Geometry: final body of the model. Coordinates: model frame, mm. Round coordinates to 2 decimals unless told otherwise and drop trailing zeros. Loops run counter-clockwise (first coordinate to the right, second up) from the corner with the lowest first, then second, coordinate; pieces in that order, holes last. Notation, with made-up numbers: (19.25, 2.25) -> (50.25, 2.25) arc R37 cw to (50.25, 38.25) -> close; hole circle Ø1 at (-6, 28). An arc over 180 degrees is marked (long way). Answer in a Markdown table with one row per item.
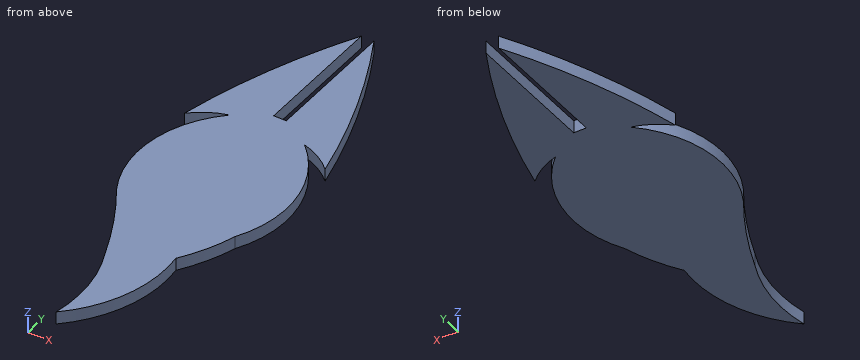
```python
from build123d import *

# Parameters (mm, degrees)
BOSS_EXTRUDE1_DEPTH = 1.524


with BuildPart() as part:
    # Sketch1 → Boss-Extrude1 (new body)
    with BuildSketch(Plane.XY):
        with BuildLine():
            Line((-1.524, -34.676201819), (0, -34.676201819))
            Line((0, -34.676201819), (0, -18.581601914))
            ThreePointArc((0, -18.581601914), (4.586568454, -28.671218755), (7.766480304, -39.288428313))
            ThreePointArc((7.766480304, -39.288428313), (5.922115133, -37.899455621), (3.784796816, -37.026072296))
            ThreePointArc((3.784796816, -37.026072296), (8.024285986, -44.938100791), (6.429295491, -53.771529834))
            ThreePointArc((6.429295491, -53.771529834), (5.182840175, -57.065431108), (3.445514823, -60.128948218))
            ThreePointArc((3.445514823, -60.128948218), (2.639499088, -67.873650649), (-1.687439347, -74.347264855))
            ThreePointArc((-1.687439347, -74.347264855), (-1.444255212, -68.732462045), (-3.001469179, -63.332440397))
            ThreePointArc((-3.001469179, -63.332440397), (-5.223476479, -58.420481145), (-7.953295491, -53.771529834))
            ThreePointArc((-7.953295491, -53.771529834), (-9.548285986, -44.938100791), (-5.308796816, -37.026072296))
            ThreePointArc((-5.308796816, -37.026072296), (-7.446115133, -37.899455621), (-9.290480304, -39.288428313))
            ThreePointArc((-9.290480304, -39.288428313), (-6.110568454, -28.671218755), (-1.524, -18.581601914))
            Line((-1.524, -18.581601914), (-1.524, -34.676201819))
        make_face()
    extrude(amount=BOSS_EXTRUDE1_DEPTH)


solid = part.part
```
Item 1: First-contact query: P1, Ø0.8, axis at y = -26.5, z = 0.5, coming from the -X side. Flat tip, straight axial feed; report the tip coordinate or a pass-through.
Ans:
| item | result |
|---|---|
| P1 | x = -5.42 |
Item 2: Ray query, L1, parallel to X at y = -37.5, z = 1.3; L2, parallel to X at y = -26, z = 0.5; L3, parallel to X at y = -24.5, z = 1.45. Return the intervals inside material, ascending.
Ans:
| item | result |
|---|---|
| L1 | -8.86 to -6.65, -5.8 to 4.27, 5.13 to 7.34 |
| L2 | -5.05 to -1.52, 0 to 3.53 |
| L3 | -4.41 to -1.52, 0 to 2.89 |
Item 3: Section query C-C, the plane z = 0.9. Output: boundary loops of the cut face in (x, y), and give its area (3 significant figures).
Ans:
| item | result |
|---|---|
| outline | (-9.29, -39.29) arc R8.99 cw to (-5.31, -37.03) arc R13.64 ccw to (-7.95, -53.77) arc R50.82 cw to (-3, -63.33) arc R17.42 cw to (-1.69, -74.35) arc R16.2 ccw to (3.45, -60.13) arc R22.87 ccw to (6.43, -53.77) arc R13.64 ccw to (3.78, -37.03) arc R8.99 cw to (7.77, -39.29) arc R81.76 ccw to (0, -18.58) -> (0, -34.68) -> (-1.52, -34.68) -> (-1.52, -18.58) arc R81.76 ccw to start |
| area | 557 mm2 |
Item 4: Section query A-A, the plane y = -32. Output: boundary loops of the cut face in (x, z).
Ans:
| item | result |
|---|---|
| outline | (-7.28, 0) -> (-1.52, 0) -> (-1.52, 1.52) -> (-7.28, 1.52) -> close; (0, 0) -> (5.75, 0) -> (5.75, 1.52) -> (0, 1.52) -> close |
Item 5: Section query B-B, the plane x = 7. Output: boundary loops of the cut face in (y, z), and give its area (3 significant figures).
Ans:
| item | result |
|---|---|
| outline | (-52.64, 0) -> (-41.49, 0) -> (-41.49, 1.52) -> (-52.64, 1.52) -> close; (-38.62, 0) -> (-36.19, 0) -> (-36.19, 1.52) -> (-38.62, 1.52) -> close |
| area | 20.7 mm2 |
Item 6: Section query D-D, the plane y = -69.5. Output: boundary loops of the cut face in (x, z), and give its area (3 significant figures).
Ans:
| item | result |
|---|---|
| outline | (-1.37, 0) -> (1.95, 0) -> (1.95, 1.52) -> (-1.37, 1.52) -> close |
| area | 5.06 mm2 |
